from build123d import *

# Parameters (mm, degrees)
SKETCH1_W           = 160
SKETCH1_H           = 160
SKETCH1_W_2         = 152
SKETCH1_H_2         = 152
BOSS_EXTRUDE1_DEPTH = 52
SKETCH2_W           = 160
SKETCH2_H           = 160
BOSS_EXTRUDE2_DEPTH = 5
SKETCH3_R           = 1.42
CUT_EXTRUDE1_DEPTH  = 10
SKETCH4_W           = 152
SKETCH4_H           = 152
CUT_EXTRUDE2_DEPTH  = 2.5
FILLET1_R           = 10
FILLET2_R           = 10
SKETCH5_R           = 3
CUT_EXTRUDE3_DEPTH  = 2
SKETCH7_W           = 25
SKETCH7_H           = 14.209603119
CUT_EXTRUDE4_DEPTH  = 10


with BuildPart() as part:
    # Sketch1 → Boss-Extrude1 (new body)
    # profile 1 of 5: a face of its own
    with BuildSketch(Plane(origin=(0, 0, 0), x_dir=(1, 0, 0), z_dir=(0, 1, 0))):
        Rectangle(SKETCH1_W, SKETCH1_H)
        Rectangle(SKETCH1_W_2, SKETCH1_H_2, mode=Mode.SUBTRACT)
    # profile 2 of 5: a face of its own
    with BuildSketch(Plane(origin=(0, 0, 0), x_dir=(1, 0, 0), z_dir=(0, 1, 0))):
        Polygon((-61.150757595, 76), (-76, 61.150757595), (-76, 58.32233047), (-58.32233047, 76), align=None)
    # profile 3 of 5: a face of its own
    with BuildSketch(Plane(origin=(0, 0, 0), x_dir=(1, 0, 0), z_dir=(0, 1, 0))):
        Polygon((-58.32233047, -76), (-76, -58.32233047), (-76, -61.150757595), (-61.150757595, -76), align=None)
    # profile 4 of 5: a face of its own
    with BuildSketch(Plane(origin=(0, 0, 0), x_dir=(1, 0, 0), z_dir=(0, 1, 0))):
        Polygon((76, -58.32233047), (58.32233047, -76), (61.150757595, -76), (76, -61.150757595), align=None)
    # profile 5 of 5: a face of its own
    with BuildSketch(Plane(origin=(0, 0, 0), x_dir=(1, 0, 0), z_dir=(0, 1, 0))):
        Polygon((61.150757595, 76), (58.32233047, 76), (76, 58.32233047), (76, 61.150757595), align=None)
    extrude(amount=BOSS_EXTRUDE1_DEPTH)

    # Sketch2 → Boss-Extrude2 (add)
    with BuildSketch(Plane(origin=(0, 0, 0), x_dir=(1, 0, 0), z_dir=(0, 1, 0))):
        Rectangle(SKETCH2_W, SKETCH2_H)
    extrude(amount=BOSS_EXTRUDE2_DEPTH)

    # Sketch3 → Cut-Extrude1 (cut)
    with BuildSketch(Plane(origin=(0, 5, 0), x_dir=(1, 0, 0), z_dir=(0, 1, 0))):
        with Locations(Location((-55, 55, 0), (0, 0, 270))):
            Circle(SKETCH3_R)
        with Locations(Location((55, 55, 0), (0, 0, 270))):
            Circle(SKETCH3_R)
        with Locations(Location((55, -55, 0), (0, 0, 270))):
            Circle(SKETCH3_R)
        with Locations(Location((-55, -55, 0), (0, 0, 270))):
            Circle(SKETCH3_R)
        with Locations(Location((0, 40, 0), (0, 0, 270))):
            Circle(SKETCH3_R)
        with Locations(Location((40, 0, 0), (0, 0, 270))):
            Circle(SKETCH3_R)
        with Locations(Location((0, -40, 0), (0, 0, 270))):
            Circle(SKETCH3_R)
        with Locations(Location((-40, 0, 0), (0, 0, 270))):
            Circle(SKETCH3_R)
    extrude(amount=-CUT_EXTRUDE1_DEPTH, mode=Mode.SUBTRACT)

    # Sketch4 → Cut-Extrude2 (cut)
    with BuildSketch(Plane(origin=(0, 52, 0), x_dir=(1, 0, 0), z_dir=(0, 1, 0))):
        Rectangle(SKETCH4_W, SKETCH4_H)
    extrude(amount=-CUT_EXTRUDE2_DEPTH, mode=Mode.SUBTRACT)

    # Fillet1
    fillet1_edges = [part.edges().sort_by_distance(p)[0] for p in [
        (-80, 26, 80),
        (-80, 26, -80),
        (80, 26, -80),
        (80, 26, 80),
    ]]
    fillet(fillet1_edges, radius=FILLET1_R)

    # Fillet2
    fillet2_edges = [part.edges().sort_by_distance(p)[0] for p in [
        (-76, 28.5, 76),
        (-76, 28.5, -76),
        (76, 28.5, 76),
        (76, 28.5, -76),
    ]]
    fillet(fillet2_edges, radius=FILLET2_R)

    # Sketch5 → Cut-Extrude3 (cut)
    with BuildSketch(Plane.XZ):
        with Locations(Location((-55, 55, 0), (0, 0, 270))):
            Circle(SKETCH5_R)
        with Locations(Location((55, 55, 0), (0, 0, 270))):
            Circle(SKETCH5_R)
        with Locations(Location((55, -55, 0), (0, 0, 270))):
            Circle(SKETCH5_R)
        with Locations(Location((-55, -55, 0), (0, 0, 270))):
            Circle(SKETCH5_R)
        with Locations(Location((0, 40, 0), (0, 0, 270))):
            Circle(SKETCH5_R)
        with Locations(Location((-40, 0, 0), (0, 0, 270))):
            Circle(SKETCH5_R)
        with Locations(Location((0, -40, 0), (0, 0, 270))):
            Circle(SKETCH5_R)
        with Locations(Location((40, 0, 0), (0, 0, 270))):
            Circle(SKETCH5_R)
    extrude(amount=-CUT_EXTRUDE3_DEPTH, mode=Mode.SUBTRACT)

    # Sketch7 → Cut-Extrude4 (cut)
    with BuildSketch(Plane.XY.offset(80)):
        with Locations((0, 12.10480156)):
            Rectangle(SKETCH7_W, SKETCH7_H)
    extrude(amount=-CUT_EXTRUDE4_DEPTH, mode=Mode.SUBTRACT)


solid = part.part
Can you work these out from the model? Positions are in its coordinate system, mm. A direction names the side the tool comes from. Give positions to 0.01 mm unless a question says otherwise; leave off trailing zeros. Loops run counter-clockwise (first coordinate to the right, second up) from the corner with the lowest first, then second, coordinate; pieces in that order, holes last. Notation, with made-up numbers: (81, 34.5) - (95, 34.5) arc R21 cw to (95, 46.5) - close; hole circle Ø8 at (32.5, -38.5). An arc over 180 degrees is marked (long way). Answer as a JSON object with one key per item and string values.
Q1. Imagine slicing it at C-C on z = 46.5. Write out the boundary of the cut face in (x, y), plus the area to 3 significant figures.
Geometry says:
{"outline": "(-80, 0) - (80, 0) - (80, 52) - (76, 52) - (76, 5) - (-76, 5) - (-76, 52) - (-80, 52) - close", "area": "1,180 mm²"}
Q2. Imagine slicing it at B-B on x = 47.5. Write out the boundary of the cut face in (y, z), plus the area to 3 significant figures.
Geometry says:
{"outline": "(0, -80) - (52, -80) - (52, -76) - (5, -76) - (5, 76) - (52, 76) - (52, 80) - (0, 80) - close", "area": "1,180 mm²"}
Q3. Will these pins go through, and if not, where does the flat tip stop? P1, Ø1.7, axis at x = -55, z = 55, coming from the +Y side; P2, Ø1, axis at x = -33.5, z = -6.5, coming from the +Y side; P3, Ø3, axis at x = -55, z = -54.5, coming from the -Y side.
Geometry says:
{"P1": "through", "P2": "y = 5", "P3": "y = 2"}
Q4. If I drill on L1, parallel to X at y = 0.75, z = 55; L2, parallel to X at y = 3, z = -55; L3, parallel to X at y = 38, z = 14.5, over which ranges is the centre line in solid material (lowest first)?
Geometry says:
{"L1": "-80 to -58, -52 to 52, 58 to 80", "L2": "-80 to -56.42, -53.58 to 53.58, 56.42 to 80", "L3": "-80 to -76, 76 to 80"}
Q5. If we mould it in two halves opening along Y, with no side actions, what happens to faces 1 (the flat face through (-12.5, 12, 78)), 2 (the flat face through (0, 52, 77)), 3 (the cylindrical face through (0, 1, 43))? For each: pulls with the +Y half, pulls with the -Y half, needs draft (parallel to the pull), parting line crosses it, or undercut.
Geometry says:
{"face 1": "undercut", "face 2": "pulls with the +Y half", "face 3": "needs draft"}
Q6. Imagine slicing it at A-A on y = 30.5. Give the number of separate pieces and of enclosed holes in the cut face, plus the area to 3 significant figures.
Geometry says:
{"separate pieces": "1", "enclosed holes": "5", "area": "2,680 mm²"}
Q7. Which directions (+Z, -Z, +X, -X, +Y, -Y) give clear straight access to the entire face, cutting with the end or side of a thin tool? Please do faces 4 (the cylindrical face through (77.15, 26.36, 76.99)), 5 (the flat face through (-67.28, 26.94, -67.04)), 6 (the cylindrical face through (57.03, 0.99, -52.79)).
Geometry says:
{"face 4": "+Z, +X, +Y, -Y", "face 5": "+Y", "face 6": "-Y"}
